from build123d import *

# Parameters (mm, degrees)
SKETCH1_W          = 38.1
SKETCH1_H          = 38.1
MAIN_BODY_DEPTH    = 40.64
HOLLOW_IT_T        = -2.54
SKETCH3_R          = 3.81
NIBBLE_NO_1_DEPTH  = 12.7
NIBBLE_START       = 12.7
SKETCH4_R          = 3.81
NIBBLE_NO_2_DEPTH  = 12.7
SKETCH5_W          = 1.27
SKETCH5_H          = 3.81
FLAG_DEPTH         = 0.254
SKETCH2_R          = 3.81
NIBBLE_HOLES_DEPTH = 69.261761624


with BuildPart() as part:
    # Sketch1 → main body (new body)
    with BuildSketch(Plane.XY):
        Rectangle(SKETCH1_W, SKETCH1_H)
    extrude(amount=MAIN_BODY_DEPTH)

    # hollow it
    hollow_it_openings = [part.faces().sort_by_distance(p)[0] for p in [
        (0, 19.05, 20.32),
    ]]
    offset(amount=HOLLOW_IT_T, openings=hollow_it_openings, kind=Kind.INTERSECTION)

    # Sketch3 → nibble no 1 (add)
    with BuildSketch(Plane.XY.offset(40.64)):
        with Locations(Location((0, 0, 0), (0, 0, 180))):
            Circle(SKETCH3_R)
    extrude(amount=NIBBLE_NO_1_DEPTH)

    # Sketch4 → nibble no 2 (add)
    with BuildSketch(Plane(origin=(0, 0, 0), x_dir=(-1, 0, 0), z_dir=(0, 0, -1)).offset(NIBBLE_START)):
        Circle(SKETCH4_R)
    extrude(amount=-NIBBLE_NO_2_DEPTH)

    # Sketch5 → flag (add)
    with BuildSketch(Plane(origin=(0, 0, 0), x_dir=(-1, 0, 0), z_dir=(0, -1, 0))):
        with Locations((-0.18666561, 6.353298227)):
            Rectangle(SKETCH5_W, SKETCH5_H)
    extrude(amount=FLAG_DEPTH)

    # Sketch2 → nibble holes (cut, through all)
    with BuildSketch(Plane(origin=(19.05, 0, 0), x_dir=(0, 0, -1), z_dir=(1, 0, 0))):
        with Locations((-20.32, 2.54)):
            Circle(SKETCH2_R)
    extrude(amount=-NIBBLE_HOLES_DEPTH, mode=Mode.SUBTRACT)


solid = part.part
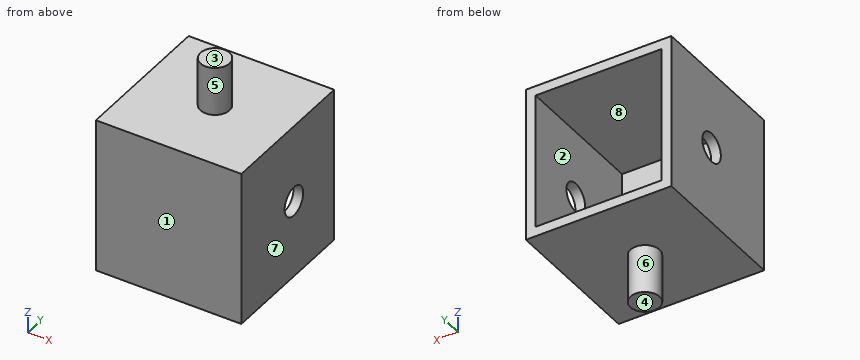
The listing builds one solid part. Answer for the finished solid, in the listing's coordinates (mm). Face numbers are marked on the shaded views. A direction names the side the tool comes from. Coordinates: 2 decimals unless noted, no trailing zeros. Loops run counter-clockwise (first coordinate to the right, second up) from the corner with the lowest first, then second, coordinate; pieces in that order, holes last.
1) Find section B-B on y = 0. Write down the section's boundary in (x, z), then the cut area to 3 significant figures.
2) Determine the mould class of the marked faces 1, 2 and 3 for opening direction Z: pulls with the +Z half, pulls with the -Z half, needs draft (parallel to the pull), parting line crosses it, or undercut.
3) Find section D-D on y = -15.5. Write down the section's boundary in (x, z).
4) Find section A-A on z = 20.32. Write down the section's boundary in (x, y), then the cut area to 3 significant figures.
5) Find section C-C on x = -5. Write down the section's boundary in (y, z).
6) Find the intervals of material crossed by L1, parallel to X at y = -9, z = 9; L2, parallel to Z at x = -3, y = 4; L3, parallel to Y at x = 17.7, z = 20.32, in increasing order.
7) Flat-ended cylindrical pins translate along their axes: pin 1 Ø4 at (x, z) = (9.5, 26) entering from +Y; pin 2 Ø10 at (x, y) = (8, -4) entering from -Z; pin 3 Ø4 at (x, y) = (6.5, -12.5) entering from +Z. Find the tip coordinate at first contact, or state that the pin passes through.
8) A tool of negligible diameter and unlimited length cuts with its end or side. For the marked faces 4, 5, 6, 7 and 8, from which of +Z, -Z, +X, -X, +Y, -Y can it reach the whole face along a straight path? Write none if from no direction.
Values:
1. outline: (-19.05, 0) - (-3.81, 0) - (-3.81, -12.7) - (3.81, -12.7) - (3.81, 0) - (19.05, 0) - (19.05, 17.48) - (16.51, 17.48) - (16.51, 2.54) - (-16.51, 2.54) - (-16.51, 17.48) - (-19.05, 17.48) - close; (-19.05, 23.16) - (-16.51, 23.16) - (-16.51, 38.1) - (16.51, 38.1) - (16.51, 23.16) - (19.05, 23.16) - (19.05, 40.64) - (3.81, 40.64) - (3.81, 53.34) - (-3.81, 53.34) - (-3.81, 40.64) - (-19.05, 40.64) - close
1. area: 539 mm2
2. face 1: needs draft
2. face 2: undercut
2. face 3: pulls with the +Z half
3. outline: (-19.05, 0) - (19.05, 0) - (19.05, 40.64) - (-19.05, 40.64) - close; hole (-16.51, 2.54) - (16.51, 2.54) - (16.51, 38.1) - (-16.51, 38.1) - close
4. outline: (-19.05, -19.05) - (19.05, -19.05) - (19.05, -1.27) - (16.51, -1.27) - (16.51, -16.51) - (-16.51, -16.51) - (-16.51, -1.27) - (-19.05, -1.27) - close; (-19.05, 6.35) - (-16.51, 6.35) - (-16.51, 19.05) - (-19.05, 19.05) - close; (16.51, 6.35) - (19.05, 6.35) - (19.05, 19.05) - (16.51, 19.05) - close
4. area: 239 mm2
5. outline: (-19.05, 0) - (19.05, 0) - (19.05, 2.54) - (-16.51, 2.54) - (-16.51, 38.1) - (19.05, 38.1) - (19.05, 40.64) - (-19.05, 40.64) - close
6. L1: x = -19.05 to -16.51, 16.51 to 19.05
6. L2: z = 0 to 2.54, 38.1 to 40.64
6. L3: y = -19.05 to -1.27, 6.35 to 19.05
7. pin 1: stops at y = -16.51
7. pin 2: stops at z = 0
7. pin 3: stops at z = 40.64
8. face 4: -Z, +X, -X, +Y, -Y
8. face 5: +Z
8. face 6: -Z
8. face 7: +Z, -Z, +X, +Y, -Y
8. face 8: +Y
